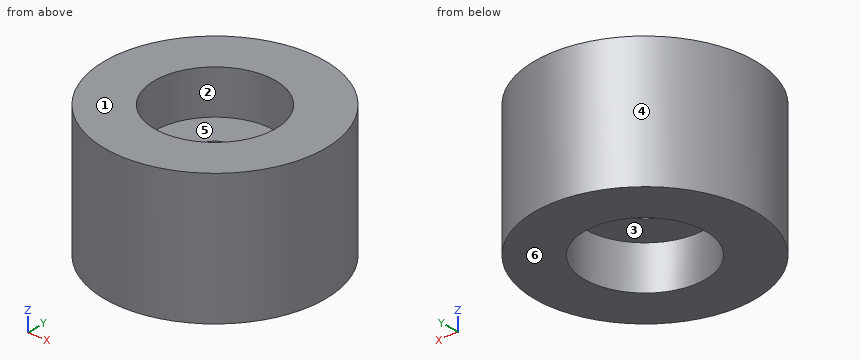
```python
from build123d import *

# Parameters (mm, degrees)
SKETCH1_R          = 20
SKETCH1_R_2        = 4
EXTRUDE1_DEPTH     = 24
SKETCH2_R          = 11
CUT_EXTRUDE1_DEPTH = 8
CUT_EXTRUDE2_START = -8
SKETCH3_R          = 11
CUT_EXTRUDE2_DEPTH = 8


with BuildPart() as part:
    # Sketch1 → Extrude1 (new body)
    with BuildSketch(Plane.XY):
        Circle(SKETCH1_R)
        Circle(SKETCH1_R_2, mode=Mode.SUBTRACT)
    extrude(amount=EXTRUDE1_DEPTH)

    # Sketch2 → Cut-Extrude1 (cut)
    with BuildSketch(Plane.XY.offset(24)):
        Circle(SKETCH2_R)
    extrude(amount=-CUT_EXTRUDE1_DEPTH, mode=Mode.SUBTRACT)

    # Sketch3 → Cut-Extrude2 (cut)
    with BuildSketch(Plane(origin=(0, 0, 0), x_dir=(-1, 0, 0), z_dir=(0, 0, -1)).offset(CUT_EXTRUDE2_START)):
        with Locations(Location((0, 0, 0), (0, 0, 180))):
            Circle(SKETCH3_R)
    extrude(amount=CUT_EXTRUDE2_DEPTH, mode=Mode.SUBTRACT)


solid = part.part
```
The model under review builds one solid part; all positions refer to its coordinate system, in mm. Face numbers are marked on the shaded views. A direction names the side the tool comes from. Round coordinates to 2 decimals unless told otherwise and drop trailing zeros. Loops run counter-clockwise (first coordinate to the right, second up) from the corner with the lowest first, then second, coordinate; pieces in that order, holes last.
1) Clearance check with flat-ended pins moving along their axes: P1, Ø17.5, axis at x = 5.5, y = 4.5, coming from the -Z side; P2, Ø6, axis at x = 4, z = 8, coming from the +Y side (3 decimals); P3, Ø8, axis at x = 0.5, z = 12, coming from the -Y side; P4, Ø20, axis at x = 0, y = 0, coming from the -Z side. State where each tip first meets the part, or that it passes through.
Values follow:
P1: stops at z = 0
P2: stops at y = 19.975
P3: stops at y = -20
P4: stops at z = 8
2) Consider section A-A on x = 0. State the section outline as (y, z) points, then the cut area to 3 significant figures.
Values follow:
outline: (-20, 0) - (-11, 0) - (-11, 8) - (-4, 8) - (-4, 16) - (-11, 16) - (-11, 24) - (-20, 24) - close; (4, 8) - (11, 8) - (11, 0) - (20, 0) - (20, 24) - (11, 24) - (11, 16) - (4, 16) - close
area: 544 mm2
3) The part is to be moulded in two halves that separate along Y. For the marked faces 4, 5 and 6, say which applies: pulls with the +Y half, pulls with the -Y half, needs draft (parallel to the pull), parting line crosses it, or undercut.
Values follow:
face 4: parting line crosses it
face 5: undercut
face 6: needs draft
4) Consider section C-C on z = 3. State the section outline as (x, y) points, then the cut area to 3 significant figures.
Values follow:
outline: circle Ø40 at (0, 0); hole circle Ø22 at (0, 0)
area: 877 mm2
5) Tool access review of the marked faces 1, 2 and 3: name each direction out of +Z, -Z, +X, -X, +Y, -Y from which nothing blocks a thin tool from reaching the whole face with its end or side.
Values follow:
face 1: +Z, +X, -X, +Y, -Y
face 2: +Z
face 3: -Z
6) Consider section D-D on y = -5.5. State the section outline as (x, z) points, then the cut area to 3 significant figures.
Values follow:
outline: (-19.23, 0) - (-9.53, 0) - (-9.53, 8) - (9.53, 8) - (9.53, 0) - (19.23, 0) - (19.23, 24) - (9.53, 24) - (9.53, 16) - (-9.53, 16) - (-9.53, 24) - (-19.23, 24) - close
area: 618 mm2
7) Wall thickness on line 1 along Y through (x, z) = (0, 5.5); line 2 along Y through (x, z) = (0, 9.75); line 3 along Z through (x, y) = (5.5, 3.5): over which ranges is each line inside the solid? List them lowest first.
Values follow:
line 1: y = -20 to -11, 11 to 20
line 2: y = -20 to -4, 4 to 20
line 3: z = 8 to 16
